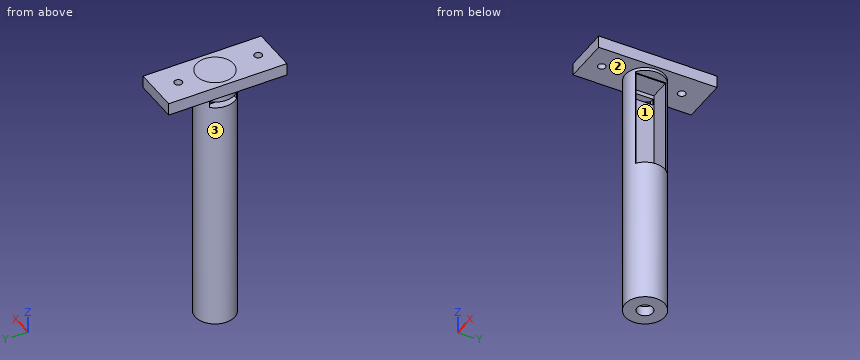
```python
from build123d import *

# Parameters (mm, degrees)
SKETCH1_R           = 8
BOSS_EXTRUDE1_DEPTH = 101.6
SKETCH2_W           = 18.519646932
SKETCH2_H           = 47.927417474
BOSS_EXTRUDE2_DEPTH = 5
SKETCH3_R           = 7.5
BOSS_EXTRUDE3_DEPTH = 0.0001
SKETCH4_R           = 1.59
CUT_EXTRUDE1_DEPTH  = 34
SKETCH7_R           = 3.185
CUT_EXTRUDE2_DEPTH  = 4
SKETCH8_W           = 8.28003219
SKETCH8_H           = 11.80237286
CUT_EXTRUDE7_DEPTH  = 96
SKETCH12_W          = 40.69032966
SKETCH12_H          = 13.123197876
CUT_EXTRUDE8_DEPTH  = 35
SKETCH13_W          = 2.556138798
SKETCH13_H          = 10.974311436
CUT_EXTRUDE9_DEPTH  = 35


with BuildPart() as part:
    # Sketch1 → Boss-Extrude1 (new body)
    with BuildSketch(Plane.XY):
        Circle(SKETCH1_R)
    extrude(amount=BOSS_EXTRUDE1_DEPTH)

    # Sketch2 → Boss-Extrude2 (add)
    with BuildSketch(Plane.XY.offset(101.6)):
        Rectangle(SKETCH2_W, SKETCH2_H)
    extrude(amount=BOSS_EXTRUDE2_DEPTH)

    # Sketch3 → Boss-Extrude3 (add)
    with BuildSketch(Plane.XY.offset(106.6)):
        Circle(SKETCH3_R)
    extrude(amount=BOSS_EXTRUDE3_DEPTH)

    # Sketch4 → Cut-Extrude1 (cut)
    with BuildSketch(Plane(origin=(0, 0, 101.6), x_dir=(-1, 0, 0), z_dir=(0, 0, -1))):
        with Locations((0, 14.883091948)):
            Circle(SKETCH4_R)
        with Locations((0, -17.523878239)):
            Circle(SKETCH4_R)
    extrude(amount=-CUT_EXTRUDE1_DEPTH, mode=Mode.SUBTRACT)

    # Sketch7 → Cut-Extrude2 (cut)
    with BuildSketch(Plane(origin=(0, 0, 0), x_dir=(-1, 0, 0), z_dir=(0, 0, -1))):
        Circle(SKETCH7_R)
    extrude(amount=-CUT_EXTRUDE2_DEPTH, mode=Mode.SUBTRACT)

    # Sketch8 → Cut-Extrude7 (cut)
    with BuildSketch(Plane(origin=(0, 0, 4), x_dir=(-1, 0, 0), z_dir=(0, 0, -1))):
        Rectangle(SKETCH8_W, SKETCH8_H)
    extrude(amount=-CUT_EXTRUDE7_DEPTH, mode=Mode.SUBTRACT)

    # Sketch12 → Cut-Extrude8 (cut)
    with BuildSketch(Plane.ZY.offset(-4.140016095)):
        with Locations((80.002136868, 0.118820051)):
            Rectangle(SKETCH12_W, SKETCH12_H)
    extrude(amount=-CUT_EXTRUDE8_DEPTH, mode=Mode.SUBTRACT)

    # Sketch13 → Cut-Extrude9 (cut)
    with BuildSketch(Plane(origin=(-4.140016095, 0, 0), x_dir=(0, 0, -1), z_dir=(1, 0, 0))):
        with Locations((-97.09530972, 0)):
            Rectangle(SKETCH13_W, SKETCH13_H)
    extrude(amount=-CUT_EXTRUDE9_DEPTH, mode=Mode.SUBTRACT)


solid = part.part
```
The model under review builds one solid part; all positions refer to its coordinate system, in mm. Face numbers are marked on the shaded views. Coordinates: 2 decimals unless noted, no trailing zeros. Order: outer loops, then holes, each group sorted by start corner. A loop starts at its lowest first (then second) coordinate and runs counter-clockwise, first axis right, second up. Notation, with made-up numbers: M 29,14 L 75,14 A25 ccw 75,36 Z; hole C 3,37.25 d11. An arc over 180 degrees is marked long. One line per question, with ' | ' between items.
(1) The part is to be moulded in two halves that separate along X. For the marked faces 1, 2 and 3, say which applies: +X half, -X half, draft (parallel to the pull), parting line (faces both ways), or undercut.
Geometry results:
face 1: undercut | face 2: draft | face 3: parting line
(2) Add section A-A, the plane x = 0. State how many separate pieces and enclosed holes the cut face has, then the cut area to 3 significant figures.
Geometry results:
separate pieces: 3 | enclosed holes: 0 | area: 675 mm²
(3) Insertion check: pin 1 (6.5 mm diameter, centred on x = 0.5, z = 64, fed in from -Y); pin 2 (2 mm diameter, centred on x = -2, z = 68.5, fed in from -Y); pin 3 (3 mm diameter, centred on x = -7, z = 13, fed in from +Y). Each pin has a flat end and moves straight along its axis. Give the tip position at first contact, or say it passes through.
Geometry results:
pin 1: stops at y = -8 | pin 2: stops at y = -7.94 | pin 3: stops at y = 5.81
(4) Add section C-C, the plane z = 61.5. Write out the cut boundary in (x, y).
Geometry results:
outline: M -4.14,-5.9 L -4.14,5.9 L 4.14,5.9 L 4.14,6.68 L 4.4,6.68 A8 ccw long 4.74,-6.44 L 4.14,-6.44 L 4.14,-5.9 Z
(5) Add section D-D, the plane z = 8. Write out the cut boundary in (x, y).
Geometry results:
outline: C 0,0 d16; hole M -4.14,-5.9 L 4.14,-5.9 L 4.14,5.9 L -4.14,5.9 Z
(6) For probe 1 along Y at (x, z) = (0, 104.7); probe 2 along Z at (x, y) = (2.75, 2); probe 3 along Y at (x, z) = (0, 2.35) (3 decimals), list the stretches that pass through material, from the lowest coordinate up. Write a range as from..to.
Geometry results:
probe 1: y = -23.96..-19.11, -15.93..13.29, 16.47..23.96 | probe 2: z = 0..4, 100..106.6 | probe 3: y = -8..-3.185, 3.185..8
